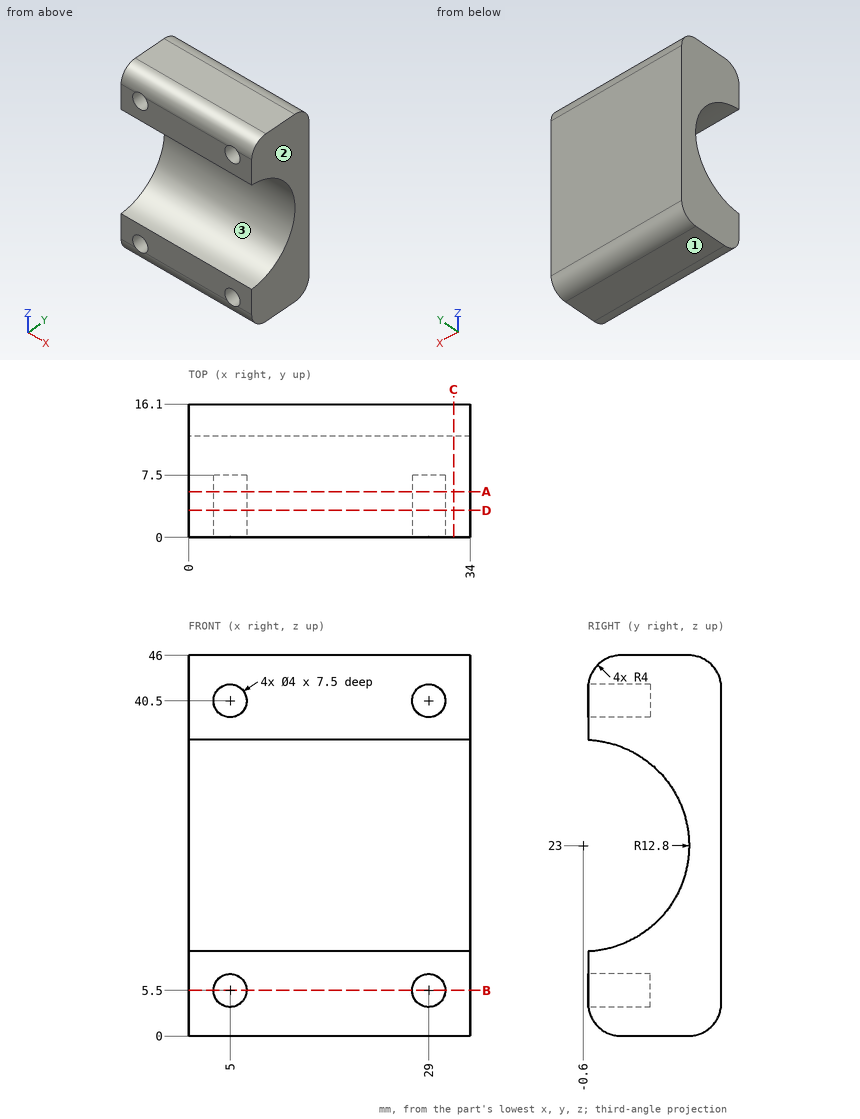
For this review, use the dimensioned drawing (mm, ordinates from the lowest corner) and the shaded views. Coordinates: 2 decimals unless noted, no trailing zeros. Loops run counter-clockwise (first coordinate to the right, second up) from the corner with the lowest first, then second, coordinate; pieces in that order, holes last. Notation, with made-up numbers: (30, 3.25) - (80, 3.25) arc R35 ccw to (80, 41.25) - close; hole circle Ø7 at (-26, 82). An arc over 180 degrees is marked (long way). Use one line per item in the form item = value. Start each with the question number.
1) Take a section at C-C (x = 32). State the section outline as (y, z) points.
2) To check wall thickness, follow probe 1 along X at (y, z) = (4.75, 5.5); probe 2 along Z at (x, y) = (28, 6.75); probe 3 along Z at (x, y) = (3.5, 6.5). State the ranges of each line that lie inside material, in increasing order. Write a range as from..to.
3) Take a section at B-B (z = 5.5). State the section outline as (x, y) points, plus the area to 3 significant figures.
4) Take a section at A-A (y = 5.5). State the section outline as (x, z) points.
5) Draft analysis for pull direction Z (two halves, no side actions). For the marked faces 1, 2 and 3, state which applies: released by +Z, released by -Z, zero draft, split by the parting line, or undercut.
6) For pin 1 (3 mm diameter, centred on x = 7.5, z = 22, fed in from -Y); pin 2 (1.5 mm diameter, centred on x = 20.5, y = 3, fed in from +Z); pin 3 (2 mm diameter, centred on x = 30.5, y = 14.5, fed in from +Z), all flat-tipped, find the tip position at first contact; note any pin that passes through.
7) Take a section at D-D (y = 3.25). State the section outline as (x, z) points.
From the geometry:
q1.outline = (0, 4) arc R4 ccw to (4, 0) - (12.1, 0) arc R4 ccw to (16.1, 4) - (16.1, 42) arc R4 ccw to (12.1, 46) - (4, 46) arc R4 ccw to (0, 42) - (0, 35.79) arc R12.8 cw to (0, 10.21) - close
q2.probe_1 = 0..3, 7..27, 31..34
q2.probe_2 = 0..3.77, 7.23..12.52, 33.48..38.77, 42.23..46
q2.probe_3 = 0..4.18, 6.82..12.35, 33.65..39.18, 41.82..46
q3.outline = (0, 0) - (3, 0) - (3, 7.5) - (7, 7.5) - (7, 0) - (27, 0) - (27, 7.5) - (31, 7.5) - (31, 0) - (34, 0) - (34, 16.1) - (0, 16.1) - close
q3.area = 487 mm2
q4.outline = (0, 0) - (34, 0) - (34, 11.75) - (0, 11.75) - close; (0, 34.25) - (34, 34.25) - (34, 46) - (0, 46) - close; hole circle Ø4 at (5, 5.5); hole circle Ø4 at (5, 40.5); hole circle Ø4 at (29, 5.5); hole circle Ø4 at (29, 40.5)
q5.face_1 = released by -Z
q5.face_2 = zero draft
q5.face_3 = undercut
q6.pin_1 = 11.95
q6.pin_2 = 45.99
q6.pin_3 = 45.75
q7.outline = (0, 0.07) - (34, 0.07) - (34, 10.79) - (0, 10.79) - close; (0, 35.21) - (34, 35.21) - (34, 45.93) - (0, 45.93) - close; hole circle Ø4 at (5, 5.5); hole circle Ø4 at (5, 40.5); hole circle Ø4 at (29, 5.5); hole circle Ø4 at (29, 40.5)
